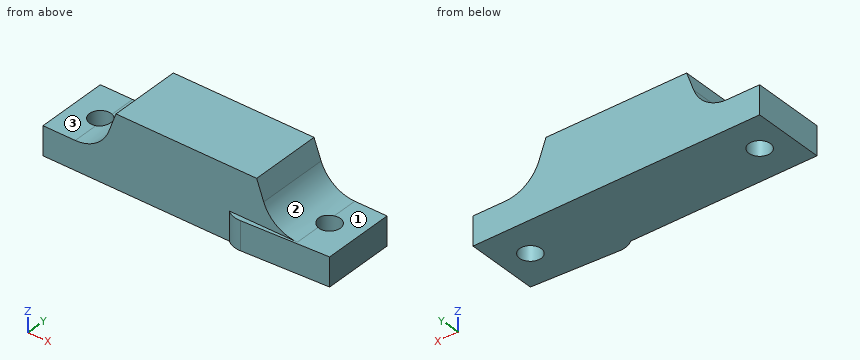
```python
from build123d import *

# Parameters (mm, degrees)
F1_DEPTH    = 5
F2_R        = 5
F3_R        = 1.5
F4_DEPTH    = 25
F6_DEPTH    = 4
F7_T1_DEPTH = 14.4192067173


# Not quite as in the source:
# - a fillet or chamfer that OpenCascade refuses, or shapes differently, is made with other operations: its cross-section is extruded or revolved along the edge and cut away or added


with BuildPart() as f1:
    # F0 (on Front) → F1 (new body, symmetric)
    with BuildSketch(Plane.XZ):
        Polygon((0, 4), (0, 0), (40, 0), (40, 4), (32, 4), (29.8161785944, 10), (10.1838214056, 10), (8, 4), align=None)
    extrude(amount=F1_DEPTH, both=True)

    # F2
    f2_edges = [f1.edges().sort_by_distance(p)[0] for p in [
        (32, 0, 4),
        (8, 0, 4),
    ]]
    fillet(f2_edges, radius=F2_R)

    # F3 (on Top) → F4 (cut)
    with BuildSketch(Plane.XY):
        with Locations((4, 0)):
            Circle(F3_R)
        with Locations((36, 0)):
            Circle(F3_R)
    extrude(amount=F4_DEPTH, mode=Mode.SUBTRACT)

    # F5 (on Top) → F6 (join)
    with BuildSketch(Plane.XY):
        Polygon((26, -5.8), (40, -5), (26, -5), align=None)
    extrude(amount=F6_DEPTH)

    # F7: fillet of radius 3 on 1 edges, made by hand

    # F7_s2 → F7_t1 (cut)
    with BuildSketch(Plane.XY.offset(-5.2096033586)):
        with BuildLine():
            ThreePointArc((26, -5), (26.9758794109, -5.5370959816), (28.0804474628, -5.6811172878))
            Line((28.0804474628, -5.6811172878), (26, -5.8))
            Line((26, -5.8), (26, -5))
        make_face()
    extrude(amount=F7_T1_DEPTH, mode=Mode.SUBTRACT)


solid = f1.part
```
Read the model definition and answer for the solid it produces. Units are mm, in the model's axes. Face numbers are marked on the shaded views. A direction names the side the tool comes from. Give positions to 0.01 mm unless a question says otherwise; leave off trailing zeros. Order: outer loops, then holes, each group sorted by start corner. A loop starts at its lowest first (then second) coordinate and runs counter-clockwise, first axis right, second up. Notation, with made-up numbers: (16, 45.25) -> (35, 45.25) arc R17 ccw to (35, 57.25) -> close; hole circle Ø11 at (-9.75, 58.25). An arc over 180 degrees is marked (long way). Write item = value, one per line.
1. A cutting plane is placed at D-D, the plane x = 36.5. Write down the section's boundary in (y, z).
Numbers:
outline = (-5.2, 0) -> (-1.41, 0) -> (-1.41, 4) -> (-5.2, 4) -> close; (1.41, 0) -> (5, 0) -> (5, 4) -> (1.41, 4) -> close
2. A cutting plane is placed at A-A, the plane x = 4. Write down the section's boundary in (y, z), and give its area (3 significant figures).
Numbers:
outline = (-5, 0) -> (-1.5, 0) -> (-1.5, 4) -> (-5, 4) -> close; (1.5, 0) -> (5, 0) -> (5, 4) -> (1.5, 4) -> close
area = 28.0 mm²
3. Straight lines are drawn through the part: line 1 along X through (y, z) = (0, 2.05); line 2 along Y through (x, z) = (4, 3); line 3 along X through (y, z) = (-1.25, 2.25). For each, find the intervals that lie inside material, in ascending order.
Numbers:
line_1 = 0 to 2.5, 5.5 to 34.5, 37.5 to 40
line_2 = -5 to -1.5, 1.5 to 5
line_3 = 0 to 3.17, 4.83 to 35.17, 36.83 to 40
4. For the marked faces 1, 2 and 3, determine the directions among +Z, -Z, +X, -X, +Y, -Y from which every point of the face is accessible in a straight line to the end or side of a thin tool.
Numbers:
face_1 = +Z, +X, -Y
face_2 = +Z, +X, +Y, -Y
face_3 = +Z, -X, +Y, -Y
5. A cutting plane is placed at B-B, the plane z = 1. Write down the section's boundary in (x, y), and give its area (3 significant figures).
Numbers:
outline = (0, -5) -> (26, -5) arc R3 ccw to (28.08, -5.68) -> (40, -5) -> (40, 5) -> (0, 5) -> close; hole circle Ø3 at (4, 0); hole circle Ø3 at (36, 0)
area = 391 mm²
6. Given pin 1 (1 mm diameter, centred on x = 6, y = 0, fed in from +Z); pin 2 (5 mm diameter, centred on x = 14.5, z = 3, fed in from -Y); pin 3 (1.3 mm diameter, centred on x = 2, y = -1.5, fed in from +Z), each flat-ended and moving along its own axis, determine where each tip first touches the part or whether it passes through.
Numbers:
pin_1 = 4.42
pin_2 = -5
pin_3 = 4
7. A cutting plane is placed at C-C, the plane y = 3.25. Write down the section's boundary in (x, z), and give its area (3 significant figures).
Numbers:
outline = (0, 0) -> (40, 0) -> (40, 4) -> (35.5, 4) arc R5 cw to (30.8, 7.29) -> (29.82, 10) -> (10.18, 10) -> (9.2, 7.29) arc R5 cw to (4.5, 4) -> (0, 4) -> close
area = 295 mm²
